```python
from build123d import *

# Parameters (mm, degrees)
SKETCH1_W           = 40
SKETCH1_H           = 40
BOSS_EXTRUDE1_DEPTH = 3.5
SKETCH2_R           = 1.05
CUT_EXTRUDE1_DEPTH  = 3.5
SKETCH3_W           = 40
SKETCH3_H           = 40
SKETCH3_W_2         = 38
SKETCH3_H_2         = 38
BOSS_EXTRUDE2_DEPTH = 5
FILLET1_R           = 2
SKETCH4_W           = 11
SKETCH4_H           = 6
CUT_EXTRUDE2_DEPTH  = 5
SKETCH5_W           = 15.9
SKETCH5_H           = 32.39
CUT_EXTRUDE7_DEPTH  = 2
SKETCH7_W           = 43.568171074
SKETCH7_H           = 43.096637318
CUT_EXTRUDE9_DEPTH  = 1


with BuildPart() as part:
    # Sketch1 → Boss-Extrude1 (new body)
    with BuildSketch(Plane(origin=(0, 0, 0), x_dir=(1, 0, 0), z_dir=(0, 1, 0))):
        Rectangle(SKETCH1_W, SKETCH1_H)
    extrude(amount=BOSS_EXTRUDE1_DEPTH)

    # Sketch2 → Cut-Extrude1 (cut)
    with BuildSketch(Plane(origin=(0, 3.5, 0), x_dir=(1, 0, 0), z_dir=(0, 1, 0))):
        with Locations(Location((-16.970562748, 16.970562748, 0), (0, 0, 270))):
            Circle(SKETCH2_R)
        with Locations(Location((16.970562748, 16.970562748, 0), (0, 0, 270))):
            Circle(SKETCH2_R)
        with Locations(Location((-16.970562748, -16.970562748, 0), (0, 0, 270))):
            Circle(SKETCH2_R)
        with Locations(Location((16.970562748, -16.970562748, 0), (0, 0, 270))):
            Circle(SKETCH2_R)
        with Locations(Location((-13.788582233, 13.788582233, 0), (0, 0, 270))):
            Circle(SKETCH2_R)
        with Locations(Location((13.788582233, 13.788582233, 0), (0, 0, 270))):
            Circle(SKETCH2_R)
        with Locations(Location((13.788582233, -13.788582233, 0), (0, 0, 270))):
            Circle(SKETCH2_R)
        with Locations(Location((-13.788582233, -13.788582233, 0), (0, 0, 270))):
            Circle(SKETCH2_R)
    extrude(amount=-CUT_EXTRUDE1_DEPTH, mode=Mode.SUBTRACT)

    # Sketch3 → Boss-Extrude2 (add)
    with BuildSketch(Plane(origin=(0, 3.5, 0), x_dir=(1, 0, 0), z_dir=(0, 1, 0))):
        Rectangle(SKETCH3_W, SKETCH3_H)
        Rectangle(SKETCH3_W_2, SKETCH3_H_2, mode=Mode.SUBTRACT)
    extrude(amount=BOSS_EXTRUDE2_DEPTH)

    # Fillet1
    fillet1_edges = [part.edges().sort_by_distance(p)[0] for p in [
        (20, 4.25, 20),
        (-20, 4.25, 20),
        (-20, 4.25, -20),
        (20, 4.25, -20),
    ]]
    fillet(fillet1_edges, radius=FILLET1_R)

    # Sketch4 → Cut-Extrude2 (cut)
    with BuildSketch(Plane(origin=(0, 3.5, 0), x_dir=(1, 0, 0), z_dir=(0, 1, 0))):
        with Locations((0, 13.75)):
            Rectangle(SKETCH4_W, SKETCH4_H)
    extrude(amount=-CUT_EXTRUDE2_DEPTH, mode=Mode.SUBTRACT)

    # Sketch5 → Cut-Extrude7 (cut)
    with BuildSketch(Plane.XZ):
        with BuildLine():
            Line((-7.81, 18.511021166), (7.81, 18.511021166))
            ThreePointArc((7.81, 18.511021166), (9.931320344, 17.632341509), (10.81, 15.511021166))
            Line((10.81, 15.511021166), (10.81, -16.688978834))
            ThreePointArc((10.81, -16.688978834), (9.931320344, -18.810299178), (7.81, -19.688978834))
            Line((7.81, -19.688978834), (-7.81, -19.688978834))
            ThreePointArc((-7.81, -19.688978834), (-9.931320344, -18.810299178), (-10.81, -16.688978834))
            Line((-10.81, -16.688978834), (-10.81, 15.511021166))
            ThreePointArc((-10.81, 15.511021166), (-9.931320344, 17.632341509), (-7.81, 18.511021166))
        make_face()
        with Locations((0, -0.483978834)):
            Rectangle(SKETCH5_W, SKETCH5_H, mode=Mode.SUBTRACT)
    extrude(amount=-CUT_EXTRUDE7_DEPTH, mode=Mode.SUBTRACT)

    # Sketch7 → Cut-Extrude9 (cut)
    with BuildSketch(Plane(origin=(0, 8.5, 0), x_dir=(1, 0, 0), z_dir=(0, 1, 0))):
        Rectangle(SKETCH7_W, SKETCH7_H)
    extrude(amount=-CUT_EXTRUDE9_DEPTH, mode=Mode.SUBTRACT)


solid = part.part
```
Check sheet for the modelled part. Datum: model origin and axes. Units: mm. A direction names the side the tool comes from. Round coordinates to 2 decimals unless told otherwise and drop trailing zeros. Loops run counter-clockwise (first coordinate to the right, second up) from the corner with the lowest first, then second, coordinate; pieces in that order, holes last. Notation, with made-up numbers: M 44,6 L 77,6 A26 cw 77,28 Z; hole C -14,-16.5 d11. An arc over 180 degrees is marked long. Answer as a JSON object with one key per item and string values.
1. Section check D-D (z = 11). Record the boundary of the cut face in (x, y), plus the area to 3 significant figures.
Reply:
{"outline": "M -20,0 L -10.81,0 L -10.81,2 L -7.95,2 L -7.95,0 L 7.95,0 L 7.95,2 L 10.81,2 L 10.81,0 L 20,0 L 20,7.5 L 19,7.5 L 19,3.5 L -19,3.5 L -19,7.5 L -20,7.5 Z", "area": "137 mm²"}
2. Gauge pin test, flat ends, axial feed: P1, Ø2.5, axis at x = 13.79, z = -13.79, coming from the +Y side; P2, Ø1.7, axis at x = -13.79, z = -13.79, coming from the -Y side. Record the tip position at first contact, or that the pin passes through.
Reply:
{"P1": "stops at y = 3.5", "P2": "passes through"}
3. Section check B-B (z = -12). Record the boundary of the cut face in (x, y).
Reply:
{"outline": "M -20,0 L -10.81,0 L -10.81,2 L -7.95,2 L -7.95,0 L -5.5,0 L -5.5,3.5 L -19,3.5 L -19,7.5 L -20,7.5 Z; M 5.5,0 L 7.95,0 L 7.95,2 L 10.81,2 L 10.81,0 L 20,0 L 20,7.5 L 19,7.5 L 19,3.5 L 5.5,3.5 Z"}
4. Access from +Z, -Z, +X, -X, +Y, -Y to the whole of each face (thin tool, end or side, straight path). Record for faces 1 (the flat face through (0, 5, -19)), 2 (the cylindrical face through (9.908, 0.986, 17.656)), 3 (the cylindrical face through (-17.996, 1.774, 16.743)).
Reply:
{"face 1": "+Y", "face 2": "-Y", "face 3": "+Y, -Y"}
5. Section check C-C (x = 6). Record the boundary of the cut face in (y, z), plus the area to 3 significant figures.
Reply:
{"outline": "M 0,-20 L 7.5,-20 L 7.5,-19 L 3.5,-19 L 3.5,19 L 7.5,19 L 7.5,20 L 0,20 L 0,18.51 L 2,18.51 L 2,15.71 L 0,15.71 L 0,-16.68 L 2,-16.68 L 2,-19.69 L 0,-19.69 Z", "area": "136 mm²"}
6. Section check A-A (y = 1). State how many separate pieces and enclosed holes the cut face has, plus the area to 3 significant figures.
Reply:
{"separate pieces": "2", "enclosed holes": "9", "area": "1,200 mm²"}
7. Scan lines: line 1 (Z direction, x = -2, y = 0.5); line 2 (Z direction, x = -17, y = 1.5); line 3 (X direction, y = 1.25, z = -9.5). Record each from-to range of solid material in increasing order.
Reply:
{"line 1": "z = -20 to -19.69, -10.75 to 15.71, 18.51 to 20", "line 2": "z = -20 to -18.02, -15.92 to 15.92, 18.02 to 20", "line 3": "x = -20 to -10.81, -7.95 to 7.95, 10.81 to 20"}
8. Mould release check, pull along Z, two halves, no side actions. Record for faces 4 (the flat face through (-14, 0, 0)), 5 (the cylindrical face through (12.857, 1.774, 14.273)), 6 (the flat face through (0, 4, 20)): pulls with the +Z half, pulls with the -Z half, needs draft (parallel to the pull), parting line crosses it, or undercut.
Reply:
{"face 4": "needs draft", "face 5": "undercut", "face 6": "pulls with the +Z half"}
